Geometry check sheet. Reference: the model listing, model coordinates, mm. A direction names the side the tool comes from. Give positions to 0.01 mm unless a question says otherwise; leave off trailing zeros. Write each loop counter-clockwise with the first axis right and the second up, starting at its lowest first coordinate (ties: lowest second). Pieces come first, ordered by that corner, then holes. Notation, with made-up numbers: (-28.75, 87) -> (-7.75, 87) arc R17 ccw to (-7.75, 119) -> close; hole circle Ø3 at (64, 49). An arc over 180 degrees is marked (long way). One line per item, written item: value.
from build123d import *

# Parameters (mm, degrees)
F0_W      = 131.4026266336
F0_H      = 56.0864862055
F1_DEPTH  = 60
F2_R      = 10.9077642955
F3_DEPTH  = 10
F4_R      = 10.8428026433
F5_DEPTH  = 10
F6_W      = 126.3662874699
F6_H      = 54.2550897226
F6_R      = 5.3589813308
F6_R_2    = 14.1599191497
F6_R_3    = 5.3638725935
F6_R_4    = 11.6614642788
F7_DEPTH  = 25
F8_DEPTH  = 30
F9_W      = 5.9520327486
F9_H      = 60
F10_DEPTH = 49.7
F11_R     = 11.6614642788
F12_DEPTH = 25


with BuildPart() as f1:
    # F0 (on Front) → F1 (new body)
    with BuildSketch(Plane.XZ):
        with Locations((0.6867721677, -6.2954211608)):
            Rectangle(F0_W, F0_H)
    extrude(amount=F1_DEPTH)

    # F2 (on face) → F3 (join)
    with BuildSketch(Plane.XY.offset(21.747821942)):
        with Locations((-51.6166612506, -46.0898727179)):
            Circle(F2_R)
        with Locations((-26.6166612506, -46.0898727179)):
            Circle(F2_R)
        with Locations((-1.6166612506, -46.0898727179)):
            Circle(F2_R)
        with Locations((23.3833387494, -46.0898727179)):
            Circle(F2_R)
        with Locations((48.3833387494, -46.0898727179)):
            Circle(F2_R)
    extrude(amount=F3_DEPTH)

    # F4 (on face) → F5 (join)
    with BuildSketch(Plane.XY.offset(21.747821942)):
        with Locations((-52.4114146829, -13.7527212501)):
            Circle(F4_R)
        with Locations((-27.4114146829, -13.7527212501)):
            Circle(F4_R)
        with Locations((-2.4114146829, -13.7527212501)):
            Circle(F4_R)
        with Locations((22.5885853171, -13.7527212501)):
            Circle(F4_R)
        with Locations((47.5885853171, -13.7527212501)):
            Circle(F4_R)
    extrude(amount=F5_DEPTH)

    # F6 (on face) → F7 (cut)
    with BuildSketch(Plane(origin=(0, 0, -34.3386642635), x_dir=(1, 0, 0), z_dir=(0, 0, -1))):
        with Locations((0.9156987071, 29.8746381886)):
            Rectangle(F6_W, F6_H)
        with Locations((-55.1707856357, 11.4462208003)):
            Circle(F6_R, mode=Mode.SUBTRACT)
        with Locations((-17.1707856357, 11.4462208003)):
            Circle(F6_R, mode=Mode.SUBTRACT)
        with Locations((20.8292143643, 11.4462208003)):
            Circle(F6_R, mode=Mode.SUBTRACT)
        with Locations((56.1292143643, 11.4462208003)):
            Circle(F6_R, mode=Mode.SUBTRACT)
        with Locations((-38.5763026357, 30.70631437)):
            Circle(F6_R_2, mode=Mode.SUBTRACT)
        with Locations((1.3236973643, 30.70631437)):
            Circle(F6_R_2, mode=Mode.SUBTRACT)
        with Locations((-54.7129400074, 48.989828676)):
            Circle(F6_R_3, mode=Mode.SUBTRACT)
        with Locations((-17.8129400074, 48.989828676)):
            Circle(F6_R_3, mode=Mode.SUBTRACT)
        with Locations((41.2236973643, 30.70631437)):
            Circle(F6_R_2, mode=Mode.SUBTRACT)
        with Locations((19.0870599926, 48.989828676)):
            Circle(F6_R_3, mode=Mode.SUBTRACT)
        with Locations((56.1870599926, 48.989828676)):
            Circle(F6_R_3, mode=Mode.SUBTRACT)
        with Locations((-38.5763026357, 30.70631437)):
            Circle(F6_R_4)
        with Locations((1.2236973643, 30.70631437)):
            Circle(F6_R_4)
        with Locations((41.0236973643, 30.70631437)):
            Circle(F6_R_4)
    extrude(amount=-F7_DEPTH, mode=Mode.SUBTRACT)

    # F8 (cut): faces of the model
    f8_faces = [f1.faces().sort_by_distance(p)[0] for p in [
        (-54.7129400074, -48.989828676, -34.3386642635),
        (-17.8129400074, -48.989828676, -34.3386642635),
        (19.0870599926, -48.989828676, -34.3386642635),
        (56.1870599926, -48.989828676, -34.3386642635),
        (56.1292143643, -11.4462208003, -34.3386642635),
        (20.8292143643, -11.4462208003, -34.3386642635),
        (-17.1707856357, -11.4462208003, -34.3386642635),
        (-55.1707856357, -11.4462208003, -34.3386642635),
    ]]
    extrude(f8_faces, amount=-F8_DEPTH, mode=Mode.SUBTRACT)

    # F9 (on face) → F10 (join)
    with BuildSketch(Plane.XY.offset(21.747821942)):
        with Locations((0, -30)):
            Rectangle(F9_W, F9_H)
    extrude(amount=-F10_DEPTH)

    # F11 (on face) → F12 (cut, through all)
    with BuildSketch(Plane(origin=(0, 0, -34.3386642635), x_dir=(1, 0, 0), z_dir=(0, 0, -1))):
        with Locations((1.2236973643, 30.70631437)):
            Circle(F11_R)
    extrude(amount=-F12_DEPTH, mode=Mode.SUBTRACT)


solid = f1.part
1) Sectioned sample at A-A on z = -30. Record the cut outline in (x, y), plus the area to 3 significant figures.
Verdict:
outline: (-65.01, -60) -> (66.39, -60) -> (66.39, 0) -> (-65.01, 0) -> close; circle Ø28.32 at (-38.58, -30.71); circle Ø28.32 at (1.32, -30.71); circle Ø28.32 at (41.22, -30.71); hole (-62.27, -57) -> (64.1, -57) -> (64.1, -2.75) -> (-62.27, -2.75) -> close; hole circle Ø23.32 at (-38.58, -30.71); hole circle Ø23.32 at (1.22, -30.71); hole circle Ø23.32 at (41.02, -30.71)
area: 1,640 mm^2
2) Sectioned sample at D-D on x = -43. Record the cut outline in (y, z).
Verdict:
outline: (-60, -34.34) -> (-57, -34.34) -> (-57, -9.34) -> (-44.16, -9.34) -> (-44.16, -34.34) -> (-41.5, -34.34) -> (-41.5, -9.34) -> (-19.92, -9.34) -> (-19.92, -34.34) -> (-17.26, -34.34) -> (-17.26, -9.34) -> (-2.75, -9.34) -> (-2.75, -34.34) -> (0, -34.34) -> (0, 21.75) -> (-8.37, 21.75) -> (-8.37, 31.75) -> (-19.14, 31.75) -> (-19.14, 21.75) -> (-39.4, 21.75) -> (-39.4, 31.75) -> (-52.78, 31.75) -> (-52.78, 21.75) -> (-60, 21.75) -> close
3) Sectioned sample at B-B on z = -16. Record the cut outline in (x, y) (1 decimal).
Verdict:
outline: (-65, -60) -> (66.4, -60) -> (66.4, 0) -> (-65, 0) -> close; circle Ø28.3 at (-38.6, -30.7); circle Ø28.3 at (41.2, -30.7); hole (-62.3, -57) -> (-3, -57) -> (-3, -44.2) arc R14.2 cw to (-3, -17.2) -> (-3, -2.7) -> (-62.3, -2.7) -> close; hole circle Ø23.3 at (-38.6, -30.7); hole circle Ø23.3 at (1.2, -30.7); hole (3, -57) -> (64.1, -57) -> (64.1, -2.7) -> (3, -2.7) -> (3, -16.6) arc R14.2 cw to (3, -44.8) -> close; hole circle Ø23.3 at (41, -30.7)
4) Mould release check, pull along X, two halves, no side actions. Record for faces 4 (the flat face through (0, -10, -27.952)), 5 (the flat face through (-3, -14, 31.748)): released by +X, released by -X, zero draft, split by the parting line, or undercut.
Verdict:
face 4: undercut
face 5: zero draft
5) Sectioned sample at C-C on x = 40.5. Record the cut outline in (y, z), plus the area to 3 significant figures.
Verdict:
outline: (-60, -34.34) -> (-57, -34.34) -> (-57, -9.34) -> (-44.85, -9.34) -> (-44.85, -34.34) -> (-42.36, -34.34) -> (-42.36, -9.34) -> (-19.06, -9.34) -> (-19.06, -34.34) -> (-16.56, -34.34) -> (-16.56, -9.34) -> (-2.75, -9.34) -> (-2.75, -34.34) -> (0, -34.34) -> (0, 21.75) -> (-5.55, 21.75) -> (-5.55, 31.75) -> (-21.96, 31.75) -> (-21.96, 21.75) -> (-38.55, 21.75) -> (-38.55, 31.75) -> (-53.63, 31.75) -> (-53.63, 21.75) -> (-60, 21.75) -> close
area: 2,450 mm^2
6) Tool access check on faces 1 (the cylindrical face through (15.34, -38.72, 26.68)), 2 (the flat face through (-27, -46, 31.748)), 3 (the flat face through (41, -31, -9.339)). Record the directions out of +Z, -Z, +X, -X, +Y, -Y that give a thin tool (end or side, any length) a straight path to the whole face; none if there is none.
Verdict:
face 1: +Z
face 2: +Z, +X, -X, +Y, -Y
face 3: -Z
7) Scan lines: probe 1 along Y at (x, z) = (-17.5, -7); probe 2 along X at (y, z) = (-50.5, -11); probe 3 along X at (y, z) = (-48, 22.5). Record each from-to range of solid material in increasing order.
Verdict:
probe 1: -60 to -54.34, -43.64 to -16.8, -6.1 to 0
probe 2: -65.01 to -62.27, -2.98 to 2.98, 64.1 to 66.39
probe 3: -62.36 to -40.88, -37.36 to -15.88, -12.36 to 9.12, 12.64 to 34.12, 37.64 to 59.12
8) Depth check by flat-ended pin: pin 1 Ø6.5 at (x, y) = (-17.17, -11.45) entering from -Z; pin 2 Ø3 at (x, y) = (-51, -17) entering from -Z; pin 3 Ø3 at (x, z) = (-51, 15) entering from +Y. Enter the tip coordinate at first touch or a pass-through.
Verdict:
pin 1: z = -4.34
pin 2: z = -9.34
pin 3: y = 0
